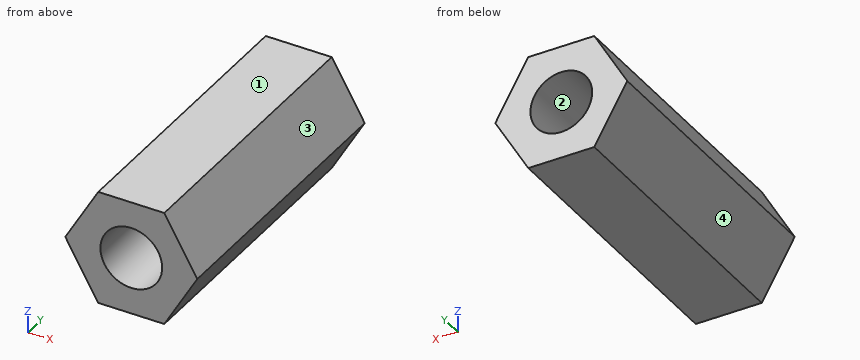
Autodesk Inventor part; units mm, degrees
ref_plane "YZ Plane" through (0, 0, 0) normal (1, 0, 0) x (0, 1, 0)
ref_plane "XZ Plane" through (0, 0, 0) normal (0, 1, 0) x (-1, 0, 0)
ref_plane "XY Plane" through (0, 0, 0) normal (0, 0, 1) x (1, 0, 0)
sketch "Sketch1" plane through (0, 0, 0) normal (0, 1, 0) x (-1, 0, 0)
  line L0 (-1.7321, -3) -> (-3.4641, 0)
  line L1 (-3.4641, 0) -> (-1.7321, 3)
  line L2 (-1.7321, 3) -> (1.7321, 3)
  line L3 (1.7321, 3) -> (3.4641, 0)
  line L4 (3.4641, 0) -> (1.7321, -3)
  line L5 (1.7321, -3) -> (-1.7321, -3)
  point P0 (0, 0)
  point P1 (0, 0)
  dimension "d0" = 3
extrude "Extrusion1" add sketch "Sketch1" along normal blind 15
sketch "Sketch2" plane through (0, 15, 0) normal (0, 1, 0) x (1, 0, 0)
  point P0 (0, 0)
hole "Hole1" at (0, 15, 0) direction (0, -1, 0) diameter 3.242 end through all
properties part number "StandoffM4x15A" material "Brass, Soft Yellow"
Design review of the part built by this model. Coordinates are the model's own, in mm. Face numbers are marked on the shaded views. Coordinates: 2 decimals unless noted, no trailing zeros. Order: outer loops, then holes, each group sorted by start corner. A loop starts at its lowest first (then second) coordinate and runs counter-clockwise, first axis right, second up. Notation, with made-up numbers: (43.5, 36.5) -> (72.5, 36.5) arc R10 ccw to (72.5, 44.5) -> close; hole circle Ø10 at (66.5, 81). An arc over 180 degrees is marked (long way). One line per item, written item: value. Start each with the question number.
Q1. Take a section at B-B, the plane x = 0. State the section outline as (y, z) points.
Q2. Take a section at A-A, the plane y = 7. State the section outline as (x, z) points.
Q3. Take a section at C-C, the plane z = 0.9. State the section outline as (x, y) points, then the cut area to 3 significant figures.
Q4. Insertion check: pin 1 Ø1 at (y, z) = (2.5, 1) entering from -X. The pin has a flat end and moves straight along its axis. Give the tip position at first contact, or say it passes through.
Q5. Mouldability with a two-part tool opening along X and no side actions: class the marked faces 1, 2, 3 and 4 as pulls with the +X half, pulls with the -X half, needs draft (parallel to the pull), parting line crosses it, or undercut.
Q6. Take a section at D-D, the plane x = 2.75. State the section outline as (y, z) points.
Q7. For probe 1 along Z at (x, y) = (0, 8.75); probe 2 along X at (y, z) = (1, 1.45); probe 3 along X at (y, z) = (2.25, -0.3), list the stretches that pass through material, from the lowest coordinate up.
Values follow:
1. outline: (0, -3) -> (15, -3) -> (15, -1.62) -> (0, -1.62) -> close; (0, 1.62) -> (15, 1.62) -> (15, 3) -> (0, 3) -> close
2. outline: (-3.46, 0) -> (-1.73, -3) -> (1.73, -3) -> (3.46, 0) -> (1.73, 3) -> (-1.73, 3) -> close; hole circle Ø3.24 at (0, 0)
3. outline: (-2.94, 0) -> (-1.35, 0) -> (-1.35, 15) -> (-2.94, 15) -> close; (1.35, 0) -> (2.94, 0) -> (2.94, 15) -> (1.35, 15) -> close
3. area: 47.9 mm2
4. pin 1: stops at x = -3.18
5. face 1: needs draft
5. face 2: undercut
5. face 3: pulls with the +X half
5. face 4: pulls with the -X half
6. outline: (0, -1.24) -> (15, -1.24) -> (15, 1.24) -> (0, 1.24) -> close
7. probe 1: z = -3 to -1.62, 1.62 to 3
7. probe 2: x = -2.63 to -0.72, 0.72 to 2.63
7. probe 3: x = -3.29 to -1.59, 1.59 to 3.29
